```python
from build123d import *

# Parameters (mm, degrees)
SKETCH1_R           = 2.54
BOSS_EXTRUDE1_DEPTH = 3.5
SKETCH2_W           = 1.5
SKETCH2_H           = 2.3
CUT_EXTRUDE1_DEPTH  = 51
SKETCH3_W           = 11.176
SKETCH3_H           = 12.2936
CUT_EXTRUDE2_DEPTH  = 3.81
SKETCH4_W           = 136.2
SKETCH4_H           = 1.4
CUT_EXTRUDE3_DEPTH  = 4.5
FILLET1_R           = 0.3


with BuildPart() as part:
    # Sketch1 → Boss-Extrude1 (new body)
    with BuildSketch(Plane.XY):
        with BuildLine():
            Line((-63.1, 2.5), (-9.742761957, 2.5))
            ThreePointArc((-9.742761957, 2.5), (0, 10.0584), (9.742761957, 2.5))
            Line((9.742761957, 2.5), (63.1, 2.5))
            Line((63.1, 2.5), (63.1, 25))
            Line((63.1, 25), (68.1, 25))
            Line((68.1, 25), (68.1, -25))
            Line((68.1, -25), (63.1, -25))
            Line((63.1, -25), (63.1, -2.5))
            Line((63.1, -2.5), (9.742761957, -2.5))
            ThreePointArc((9.742761957, -2.5), (0, -10.0584), (-9.742761957, -2.5))
            Line((-9.742761957, -2.5), (-63.1, -2.5))
            Line((-63.1, -2.5), (-63.1, -25))
            Line((-63.1, -25), (-68.1, -25))
            Line((-68.1, -25), (-68.1, 25))
            Line((-68.1, 25), (-63.1, 25))
            Line((-63.1, 25), (-63.1, 2.5))
        make_face()
        Circle(SKETCH1_R, mode=Mode.SUBTRACT)
    extrude(amount=BOSS_EXTRUDE1_DEPTH)

    # Sketch2 → Cut-Extrude1 (cut, through all)
    with BuildSketch(Plane.XZ.offset(25)):
        with Locations((67.35, 2.35)):
            Rectangle(SKETCH2_W, SKETCH2_H)
        with Locations((-67.35, 2.35)):
            Rectangle(SKETCH2_W, SKETCH2_H)
    extrude(amount=-CUT_EXTRUDE1_DEPTH, mode=Mode.SUBTRACT)

    # Sketch3 → Cut-Extrude2 (cut)
    with BuildSketch(Plane.XY.offset(3.5)):
        Rectangle(SKETCH3_W, SKETCH3_H)
    extrude(amount=-CUT_EXTRUDE2_DEPTH, mode=Mode.SUBTRACT)

    # Sketch4 → Cut-Extrude3 (cut, through all)
    with BuildSketch(Plane.XY.offset(3.5)):
        with Locations((0, 24.3)):
            Rectangle(SKETCH4_W, SKETCH4_H)
    extrude(amount=-CUT_EXTRUDE3_DEPTH, mode=Mode.SUBTRACT)

    # Fillet1
    fillet1_edges = [part.edges().sort_by_distance(p)[0] for p in [
        (-68.1, -0.7, 1.2),
        (-68.1, -0.7, 0),
    ]]
    fillet(fillet1_edges, radius=FILLET1_R)


solid = part.part
```
For this review, take the finished solid that the model builds, in its own axes (mm). A direction names the side the tool comes from. Give positions to 0.01 mm unless a question says otherwise; leave off trailing zeros. Write each loop counter-clockwise with the first axis right and the second up, starting at its lowest first coordinate (ties: lowest second). Pieces come first, ordered by that corner, then holes. Notation, with made-up numbers: M 5,31 L 24,31 A22 cw 24,61 Z; hole C 49.5,68 d1. An arc over 180 degrees is marked long. One line per item, written item: value.
1) Take a section at D-D, the plane x = -3. Write out the cut boundary in (y, z).
Results are:
outline: M -9.6,0 L -6.15,0 L -6.15,3.5 L -9.6,3.5 Z; M 6.15,0 L 9.6,0 L 9.6,3.5 L 6.15,3.5 Z
2) Take a section at C-C, the plane y = -4.5. Write out the cut boundary in (x, z).
Results are:
outline: M -68.1,0.3 A0.3 ccw -67.8,0 L -63.1,0 L -63.1,3.5 L -66.6,3.5 L -66.6,1.2 L -67.8,1.2 A0.3 ccw -68.1,0.9 Z; M -9,0 L -5.59,0 L -5.59,3.5 L -9,3.5 Z; M 5.59,0 L 9,0 L 9,3.5 L 5.59,3.5 Z; M 63.1,0 L 68.1,0 L 68.1,1.2 L 66.6,1.2 L 66.6,3.5 L 63.1,3.5 Z
3) The part is to be moulded in two halves that separate along Y. For faces 5 (the flat face through (-36, -2.5, 2)), 6 (the flat face through (5.588, 0, 2)), 7 (the flat face through (-65, 23.6, 2)), 8 (the flat face through (0, 6.147, 2)), say which applies: +Y half, -Y half, draft (parallel to the pull), parting line (faces both ways), or undercut.
Results are:
face 5: -Y half
face 6: undercut
face 7: +Y half
face 8: undercut
4) For P1, Ø1.8, axis at x = -47, z = 2.5, coming from the -Y side; P2, Ø1, axis at x = 2.5, z = 1.5, coming from the -Y side; P3, Ø0.8, axis at x = 67.5, y = 4.5, coming from the +Z side, all flat-tipped, find the tip position at first contact; note any pin that passes through.
Results are:
P1: stops at y = -2.5
P2: stops at y = -9.86
P3: stops at z = 1.2
5) Take a section at B-B, the plane z = 2.6. Write out the cut boundary in (x, y).
Results are:
outline: M -66.6,-25 L -63.1,-25 L -63.1,-2.5 L -9.74,-2.5 A10.06 ccw 9.74,-2.5 L 63.1,-2.5 L 63.1,-25 L 66.6,-25 L 66.6,23.6 L 63.1,23.6 L 63.1,2.5 L 9.74,2.5 A10.06 ccw -9.74,2.5 L -63.1,2.5 L -63.1,23.6 L -66.6,23.6 Z; hole M -5.59,-6.15 L 5.59,-6.15 L 5.59,6.15 L -5.59,6.15 Z
6) For faces 1 (the flat face through (66.6, -1, 2)), 2 (the flat face through (-66.6, -1, 2)), 3 (the flat face through (63.1, -14, 2)), 4 (the flat face through (63.1, 13, 2)), list the 3-axis set-ups (+Z, -Z, +X, -X, +Y, -Y) from which the entire face can be reached by the end or side of a thin tool; tool diameter is ignored.
Results are:
face 1: +Z, +X, +Y, -Y
face 2: +Z, -X, +Y, -Y
face 3: +Z, -Z, -Y
face 4: +Z, -Z, +Y
7) Take a section at A-A, the plane y = -14.5. Write out the cut boundary in (x, z), then the cut area to 3 significant figures.
Results are:
outline: M -68.1,0.3 A0.3 ccw -67.8,0 L -63.1,0 L -63.1,3.5 L -66.6,3.5 L -66.6,1.2 L -67.8,1.2 A0.3 ccw -68.1,0.9 Z; M 63.1,0 L 68.1,0 L 68.1,1.2 L 66.6,1.2 L 66.6,3.5 L 63.1,3.5 Z
area: 28.1 mm²
8) For line 1 (X direction, y = -13.5, z = 2.35); line 2 (X direction, y = 18, z = 0.8); line 3 (X direction, y = 6, z = 2.75), list the stretches that pass through material, from the lowest coordinate up. Write a range as from..to.
Results are:
line 1: x = -66.6..-63.1, 63.1..66.6
line 2: x = -68.1..-63.1, 63.1..68.1
line 3: x = -66.6..-63.1, -8.07..-5.59, 5.59..8.07, 63.1..66.6
